from build123d import *

# Parameters (mm, degrees)
SKETCH1_R           = 2.4892
SKETCH1_R_2         = 4.7625
BOSS_EXTRUDE1_DEPTH = 1.5875
FILLET1_R           = 3.175
SKETCH2_R           = 4.7625
SKETCH2_R_2         = 2.4892
BOSS_EXTRUDE2_DEPTH = 3.175
FILLET2_R           = 3.175


with BuildPart() as part:
    # Sketch1 → Boss-Extrude1 (new, symmetric)
    with BuildSketch(Plane(origin=(0, 0, 0), x_dir=(0, 0, -1), z_dir=(1, 0, 0))):
        with BuildLine():
            Line((6.894743879, 0), (15.875, 0))
            Line((15.875, 0), (31.75, -15.875))
            Line((31.75, -15.875), (31.75, -25.4))
            Line((31.75, -25.4), (84.1375, -25.4))
            Line((84.1375, -25.4), (84.1375, 0))
            Line((84.1375, 0), (74.6125, 0))
            ThreePointArc((74.6125, 0), (58.7375, -10.187661084), (42.8625, 0))
            Line((42.8625, 0), (38.325640303, 0))
            Line((38.325640303, 0), (31.75, 6.575640303))
            Line((31.75, 6.575640303), (31.75, 24.855256121))
            ThreePointArc((31.75, 24.855256121), (27.493760374, 31.225168873), (19.97993597, 29.730576272))
            Line((19.97993597, 29.730576272), (2.019423728, 11.77006403))
            ThreePointArc((2.019423728, 11.77006403), (0.524831127, 4.256239626), (6.894743879, 0))
        make_face()
        with Locations((6.894743879, 6.894743879)):
            Circle(SKETCH1_R, mode=Mode.SUBTRACT)
        with Locations((15.875, 15.875)):
            Circle(SKETCH1_R_2, mode=Mode.SUBTRACT)
        with Locations((24.855256121, 24.855256121)):
            Circle(SKETCH1_R, mode=Mode.SUBTRACT)
        with Locations((77.7875, -19.05)):
            Circle(SKETCH1_R, mode=Mode.SUBTRACT)
        with Locations((77.7875, -6.35)):
            Circle(SKETCH1_R, mode=Mode.SUBTRACT)
        with Locations((39.6875, -19.05)):
            Circle(SKETCH1_R, mode=Mode.SUBTRACT)
        with Locations((39.6875, -6.35)):
            Circle(SKETCH1_R, mode=Mode.SUBTRACT)
    extrude(amount=BOSS_EXTRUDE1_DEPTH, both=True)

    # Fillet1
    fillet1_edges = [part.edges().sort_by_distance(p)[0] for p in [
        (0, 0, -42.8625),
        (0, 0, -74.6125),
        (0, 0, -84.1375),
        (0, -25.4, -84.1375),
        (0, -25.4, -31.75),
        (0, -15.875, -31.75),
        (0, 0, -15.875),
        (0, 6.575640303, -31.75),
        (0, 0, -38.325640303),
    ]]
    fillet(fillet1_edges, radius=FILLET1_R)

    # Sketch2 → Boss-Extrude2 (add)
    # profile 1 of 2: a face of its own
    with BuildSketch(Plane(origin=(1.5875, 0, 0), x_dir=(0, 0, -1), z_dir=(1, 0, 0))):
        with BuildLine():
            Line((83.884613573, -25.4), (80.9625, -25.4))
            ThreePointArc((80.9625, -25.4), (83.20756403, -24.47006403), (84.1375, -22.225))
            Line((84.1375, -22.225), (84.1375, -3.175))
            ThreePointArc((84.1375, -3.175), (83.20756403, -0.92993597), (80.9625, 0))
            Line((80.9625, 0), (82.933508182, 8.621260033))
            Line((82.933508182, 8.621260033), (96.745638856, 2.180557724))
            Line((96.745638856, 2.180557724), (83.884613573, -25.4))
        make_face()
    # profile 2 of 2: a face of its own
    with BuildSketch(Plane(origin=(1.5875, 0, 0), x_dir=(0, 0, -1), z_dir=(1, 0, 0))):
        Polygon((100.377076935, 46.029113943), (114.18920761, 39.588411634), (96.745638856, 2.180557724), (82.933508182, 8.621260033), align=None)
        with Locations((98.561357896, 24.104835834)):
            Circle(SKETCH2_R, mode=Mode.SUBTRACT)
        with Locations((93.194105972, 12.594726938)):
            Circle(SKETCH2_R_2, mode=Mode.SUBTRACT)
        with Locations((103.92860982, 35.614944729)):
            Circle(SKETCH2_R_2, mode=Mode.SUBTRACT)
    extrude(amount=-BOSS_EXTRUDE2_DEPTH)

    # Fillet2
    fillet2_edges = [part.edges().sort_by_distance(p)[0] for p in [
        (0, 39.588411634, -114.18920761),
        (0, 46.029113943, -100.377076935),
        (0, 8.621260033, -82.933508182),
        (0, -25.4, -83.884613573),
        (0, 0, -80.9625),
    ]]
    fillet(fillet2_edges, radius=FILLET2_R)


solid = part.part
Geometry: final body of the model. Coordinates: model frame, mm. A direction names the side the tool comes from. Give positions to 0.01 mm unless a question says otherwise; leave off trailing zeros. Order: outer loops, then holes, each group sorted by start corner. A loop starts at its lowest first (then second) coordinate and runs counter-clockwise, first axis right, second up. Notation, with made-up numbers: (76, 37.25) -> (123, 37.25) arc R17 ccw to (123, 48.25) -> close; hole circle Ø8 at (-21, 67). An arc over 180 degrees is marked (long way). Put each result on its own line as item: value.
Q1. Section A-A, the plane y = -19.05. Return loops of the section in (x, z).
Here are the results:
outline: (-1.59, -86.85) -> (1.59, -86.85) -> (1.59, -80.28) -> (-1.59, -80.28) -> close; (-1.59, -75.3) -> (1.59, -75.3) -> (1.59, -42.18) -> (-1.59, -42.18) -> close; (-1.59, -37.2) -> (1.59, -37.2) -> (1.59, -31.75) -> (-1.59, -31.75) -> close
Q2. Draft query along Y for faces 3 (the face through (-0.022, -24.916, -83.547)), 4 (the face through (-0.02, -6.24, -37.2)), 5 (the face through (-0.02, 0.25, -38.41)), 6 (the face through (0, -20, -31.75)). Return one class per face: released by +Y, released by -Y, zero draft, split by the parting line, or undercut.
Here are the results:
face 3: released by -Y
face 4: undercut
face 5: released by +Y
face 6: zero draft
Q3. Reachability of faces 1 (the face through (-1.588, -11, -61)), 2 (the face through (0, 16, -31.75)) from +Z, -Z, +X, -X, +Y, -Y: full face, straight path, thin tool, end or side. Return the list, or none.
Here are the results:
face 1: +Z, -Z, -X, +Y, -Y
face 2: +X, -X, +Y
Q4. Pin query (flat end, axial travel): pin 1 (0.6 mm diameter, centred on x = 0, z = -77.5, fed in from +Y); pin 2 (4.5 mm diameter, centred on y = 35.61, z = -103.93, fed in from -X); pin 3 (1 mm diameter, centred on x = 0, y = 17, fed in from -Z); pin 4 (1 mm diameter, centred on x = 0, y = -16.5, fed in from +Z). Return the tip coordinate at first contact, or that it passes through.
Here are the results:
pin 1: stops at y = 0
pin 2: passes through
pin 3: stops at z = -103.89
pin 4: stops at z = -31.52
Q5. Section C-C, the plane z = -18. Return loops of the section in (x, y) (1 decimal), then the cut area to 3 significant figures.
Here are the results:
outline: (-1.6, -2.1) -> (1.6, -2.1) -> (1.6, 11.6) -> (-1.6, 11.6) -> close; (-1.6, 20.1) -> (1.6, 20.1) -> (1.6, 27.8) -> (-1.6, 27.8) -> close
area: 67.8 mm^2
Q6. Section D-D, the plane x = -0.5. Count the separate pieces of the cut face and the enclosed holes in it, then the cut area to 3 significant figures.
Here are the results:
separate pieces: 1
enclosed holes: 10
area: 2,540 mm^2
Q7. Section B-B, the plane y = -6.35. Return loops of the section in (x, z) (1 decimal), then the cut area to 3 significant figures.
Here are the results:
outline: (-1.6, -92.8) -> (1.6, -92.8) -> (1.6, -80.3) -> (-1.6, -80.3) -> close; (-1.6, -75.3) -> (1.6, -75.3) -> (1.6, -69.7) -> (-1.6, -69.7) -> close; (-1.6, -47.8) -> (1.6, -47.8) -> (1.6, -42.2) -> (-1.6, -42.2) -> close; (-1.6, -37.2) -> (1.6, -37.2) -> (1.6, -22.2) -> (-1.6, -22.2) -> close
area: 123 mm^2
Q8. Material intervals for L1, parallel to Z at x = -0.35, y = 19; L2, parallel to Z at x = -1.15, y = -20; L3, parallel to Z at x = -0.1, y = 24, sorted ascending.
Here are the results:
L1: z = -104.59 to -87.77, -31.75 to -19.47, -12.28 to -9.25
L2: z = -86.4 to -80.09, -75.49 to -41.99, -37.39 to -31.75
L3: z = -106.92 to -103.32, -93.8 to -90.1, -31.75 to -27.19, -22.52 to -14.25
